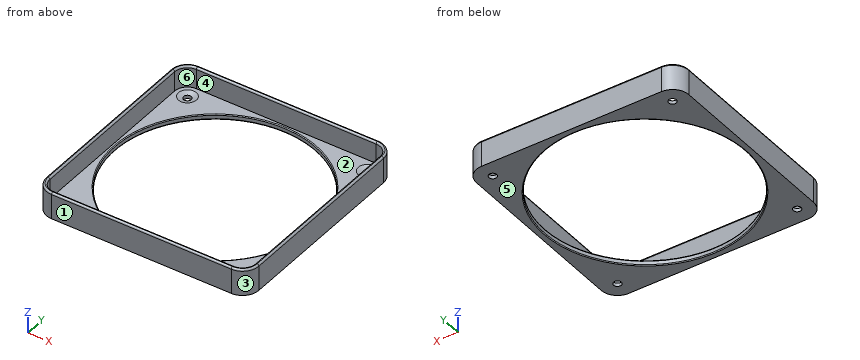
```python
from build123d import *

# Parameters (mm, degrees)
F0_R       = 2.25
F0_R_2     = 58.5
F1_DEPTH   = 3
F2_DEPTH   = 15.5
F3_R       = 0.99999
F4_SIZE2   = 3
F4_SIZE    = 1
F4_2_SIZE2 = 3
F4_2_SIZE  = 1
F4_3_SIZE2 = 3
F4_3_SIZE  = 1
F4_4_SIZE2 = 3
F4_4_SIZE  = 1
F5_R       = 0.5
F6_R       = 0.5


# Not quite as in the source:
# - a fillet or chamfer is up to 0.001 mm smaller than in the source, because OpenCascade refuses the exact size


with BuildPart() as f1:
    # F0 (on Top) → F1 (new body)
    with BuildSketch(Plane.XY):
        with BuildLine():
            Line((52.5, 60), (-52.5, 60))
            ThreePointArc((-52.5, 60), (-57.8033008589, 57.8033008589), (-60, 52.5))
            Line((-60, 52.5), (-60, -52.5))
            ThreePointArc((-60, -52.5), (-57.8033008589, -57.8033008589), (-52.5, -60))
            Line((-52.5, -60), (52.5, -60))
            ThreePointArc((52.5, -60), (57.8033008589, -57.8033008589), (60, -52.5))
            Line((60, -52.5), (60, 52.5))
            ThreePointArc((60, 52.5), (57.8033008589, 57.8033008589), (52.5, 60))
        make_face()
        with Locations((-52.5, -52.5)):
            Circle(F0_R, mode=Mode.SUBTRACT)
        with Locations((52.5, -52.5)):
            Circle(F0_R, mode=Mode.SUBTRACT)
        with Locations((-52.5, 52.5)):
            Circle(F0_R, mode=Mode.SUBTRACT)
        Circle(F0_R_2, mode=Mode.SUBTRACT)
        with Locations((52.5, 52.5)):
            Circle(F0_R, mode=Mode.SUBTRACT)
    extrude(amount=F1_DEPTH)

    # F0 (on Top) → F2 (join)
    with BuildSketch(Plane.XY):
        with BuildLine():
            ThreePointArc((-52.5, 62), (-59.2175144213, 59.2175144213), (-62, 52.5))
            Line((-62, 52.5), (-62, -52.5))
            ThreePointArc((-62, -52.5), (-59.2175144213, -59.2175144213), (-52.5, -62))
            Line((-52.5, -62), (52.5, -62))
            ThreePointArc((52.5, -62), (59.2175144213, -59.2175144213), (62, -52.5))
            Line((62, -52.5), (62, 52.5))
            ThreePointArc((62, 52.5), (59.2175144213, 59.2175144213), (52.5, 62))
            Line((52.5, 62), (-52.5, 62))
        make_face()
        with BuildLine():
            ThreePointArc((-60, 52.5), (-57.8033008589, 57.8033008589), (-52.5, 60))
            Line((-52.5, 60), (52.5, 60))
            ThreePointArc((52.5, 60), (57.8033008589, 57.8033008589), (60, 52.5))
            Line((60, 52.5), (60, -52.5))
            ThreePointArc((60, -52.5), (57.8033008589, -57.8033008589), (52.5, -60))
            Line((52.5, -60), (-52.5, -60))
            ThreePointArc((-52.5, -60), (-57.8033008589, -57.8033008589), (-60, -52.5))
            Line((-60, -52.5), (-60, 52.5))
        make_face(mode=Mode.SUBTRACT)
    extrude(amount=F2_DEPTH)

    # F3 (radius 1 in the source; OpenCascade refuses exactly that, so slightly less here)
    f3_edges = [f1.edges().sort_by_distance(p)[0] for p in [
        (-59.217514, 59.217514, 15.5),
        (-62, 0, 15.5),
        (-59.217514, -59.217514, 15.5),
        (0, -62, 15.5),
        (59.217514, -59.217514, 15.5),
        (62, 0, 15.5),
        (59.217514, 59.217514, 15.5),
        (0, 62, 15.5),
        (-57.803301, 57.803301, 15.5),
        (0, 60, 15.5),
        (57.803301, 57.803301, 15.5),
        (60, 0, 15.5),
        (57.803301, -57.803301, 15.5),
        (0, -60, 15.5),
        (-57.803301, -57.803301, 15.5),
        (-60, 0, 15.5),
    ]]
    fillet(f3_edges, radius=F3_R)

    # F4
    f4_edges = [f1.edges().sort_by_distance(p)[0] for p in [
        (-54.75, 52.5, 3),
    ]]
    f4_side = f1.faces().sort_by_distance((-54.75, 52.5, 1.5))[0]
    chamfer(f4_edges, length=F4_SIZE, length2=F4_SIZE2, reference=f4_side)

    # F4#2
    f4_2_edges = [f1.edges().sort_by_distance(p)[0] for p in [
        (-54.75, -52.5, 3),
    ]]
    f4_2_side = f1.faces().sort_by_distance((-54.75, -52.5, 1.5))[0]
    chamfer(f4_2_edges, length=F4_2_SIZE, length2=F4_2_SIZE2, reference=f4_2_side)

    # F4#3
    f4_3_edges = [f1.edges().sort_by_distance(p)[0] for p in [
        (50.25, 52.5, 3),
    ]]
    f4_3_side = f1.faces().sort_by_distance((50.25, 52.5, 1.5))[0]
    chamfer(f4_3_edges, length=F4_3_SIZE, length2=F4_3_SIZE2, reference=f4_3_side)

    # F4#4
    f4_4_edges = [f1.edges().sort_by_distance(p)[0] for p in [
        (50.25, -52.5, 3),
    ]]
    f4_4_side = f1.faces().sort_by_distance((50.25, -52.5, 1.5))[0]
    chamfer(f4_4_edges, length=F4_4_SIZE, length2=F4_4_SIZE2, reference=f4_4_side)

    # F5
    f5_edges = [f1.edges().sort_by_distance(p)[0] for p in [
        (-58.5, 0, 3),
    ]]
    fillet(f5_edges, radius=F5_R)

    # F6
    f6_edges = [f1.edges().sort_by_distance(p)[0] for p in [
        (-58.5, 0, 0),
    ]]
    fillet(f6_edges, radius=F6_R)


solid = f1.part
```
Check sheet for the modelled part. Datum: model origin and axes. Units: mm. Face numbers are marked on the shaded views. A direction names the side the tool comes from. Give positions to 0.01 mm unless a question says otherwise; leave off trailing zeros. Order: outer loops, then holes, each group sorted by start corner. A loop starts at its lowest first (then second) coordinate and runs counter-clockwise, first axis right, second up. Notation, with made-up numbers: (82.5, -13.5) -> (134.5, -13.5) arc R13 ccw to (134.5, 11.5) -> close; hole circle Ø3 at (-20, -12). An arc over 180 degrees is marked (long way). Use CSV: the item, a comma, the result in double quotes. Start each with the question number.
1) Material ranges on line 1 (Y direction, x = -6, z = 7.5); line 2 (Y direction, x = 0, z = 1.9), recorded low to high. Write a range as from..to.
2) Mould release check, pull along X, two halves, no side actions. Record for the marked faces 3, 4, 5 and 6: released by +X, released by -X, zero draft, split by the parting line, or undercut.
3) Sectioned sample at C-C, the plane z = 10.5. Record the boundary of the cut face in (x, y), plus the area to 3 significant figures.
4) Set-up check for the marked faces 1 and 2: record each of +Z, -Z, +X, -X, +Y, -Y from which the full face is reachable in a straight line by a thin tool's end or side.
5) Go/stop test with a flat-tipped pin: P1, Ø4, axis at x = 52.5, y = -52.5, coming from the -Z side. Record where the tip stops, or that it passes through.
Recorded:
1,line 1,"-62..-60, 60..62"
1,line 2,"-62..-58.5, 58.5..62"
2,face 3,"released by +X"
2,face 4,"undercut"
2,face 5,"zero draft"
2,face 6,"undercut"
3,outline,"(-62, -52.5) arc R9.5 ccw to (-52.5, -62) -> (52.5, -62) arc R9.5 ccw to (62, -52.5) -> (62, 52.5) arc R9.5 ccw to (52.5, 62) -> (-52.5, 62) arc R9.5 ccw to (-62, 52.5) -> close; hole (-60, -52.5) arc R7.5 ccw to (-52.5, -60) -> (52.5, -60) arc R7.5 ccw to (60, -52.5) -> (60, 52.5) arc R7.5 ccw to (52.5, 60) -> (-52.5, 60) arc R7.5 ccw to (-60, 52.5) -> close"
3,area,"947 mm2"
4,face 1,"+Z, -Z, +X, -X, -Y"
4,face 2,"+Z"
5,P1,"through"
